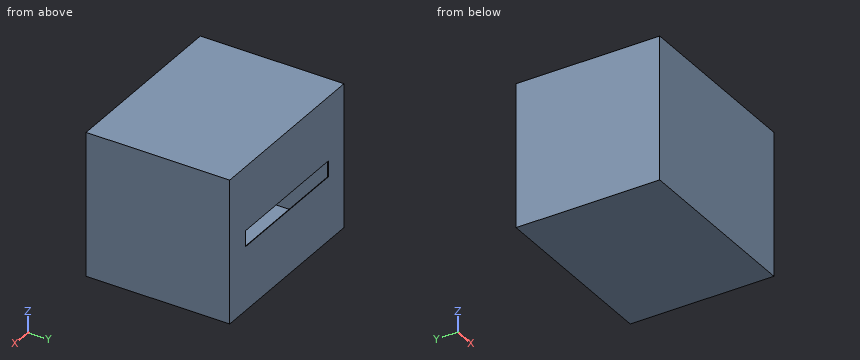
from build123d import *

# Parameters (mm, degrees)
EXTRUDE1_START     = -381
EXTRUDE1_OUTLINE_W = 965.2
EXTRUDE1_OUTLINE_H = 762
EXTRUDE1_DEPTH     = 762
SHELL1_T           = -2.54
SKETCH3_W          = 965.2
SKETCH3_H          = 762
SKETCH3_W_2        = 701.471738738
SKETCH3_H_2        = 84.826616214
EXTRUDE2_DEPTH     = 3.175


# Read off the part's stored shape, not the designer's step: Extrude1
with BuildPart() as part:
    # Extrude1 outline → Extrude1 (new body)
    with BuildSketch(Plane.XY.offset(EXTRUDE1_START)):
        with Locations((482.6, 381)):
            Rectangle(EXTRUDE1_OUTLINE_W, EXTRUDE1_OUTLINE_H)
    extrude(amount=EXTRUDE1_DEPTH)

    # Shell1
    shell1_openings = [part.faces().sort_by_distance(p)[0] for p in [
        (482.6, 762, 0),
    ]]
    offset(amount=SHELL1_T, openings=shell1_openings, kind=Kind.INTERSECTION)

    # Sketch3 → Extrude2 (add)
    with BuildSketch(Plane(origin=(0, 762, 0), x_dir=(-1, 0, 0), z_dir=(0, 1, 0))):
        with Locations((-482.6, 0)):
            Rectangle(SKETCH3_W, SKETCH3_H)
        with Locations((-482.6, 0)):
            Rectangle(SKETCH3_W_2, SKETCH3_H_2, mode=Mode.SUBTRACT)
    extrude(amount=-EXTRUDE2_DEPTH)


solid = part.part
Here's how the part is built. I have some questions about the finished solid (model axes, mm). Round coordinates to 2 decimals unless told otherwise and drop trailing zeros. Order: outer loops, then holes, each group sorted by start corner. A loop starts at its lowest first (then second) coordinate and runs counter-clockwise, first axis right, second up. Notation, with made-up numbers: M 42.25,84 L 75.25,84 A14 cw 75.25,88 Z; hole C 58,76 d2. An arc over 180 degrees is marked long. Return JSON: item names as keys, results as strings. Group by question number.
1. Please list where these lines run through material, in increasing order: probe 1 along Y at (x, z) = (416, -148.5) (3 decimals); probe 2 along Z at (x, y) = (532.5, 206.5); probe 3 along X at (y, z) = (549, 285.5).
2. If we section it at B-B on z = 283.5: List the corners of the cut face in (x, y) for me (3 decimals), then the cut area to 3 significant figures.
3. If we section it at C-C on x = 292: List the corners of the cut face in (y, z) for me (3 decimals).
4. If we section it at A-A on y = 201.5: List the corners of the cut face in (x, z) for me.
Reply:
{
 "1": {"probe 1": "0 to 2.54, 758.825 to 762", "probe 2": "-381 to -378.46, 378.46 to 381", "probe 3": "0 to 2.54, 962.66 to 965.2"},
 "2": {"outline": "M 0,0 L 965.2,0 L 965.2,762 L 0,762 Z; hole M 2.54,2.54 L 962.66,2.54 L 962.66,758.825 L 2.54,758.825 Z", "area": "9,360 mm^2"},
 "3": {"outline": "M 0,-381 L 762,-381 L 762,-42.413 L 758.825,-42.413 L 758.825,-378.46 L 2.54,-378.46 L 2.54,378.46 L 758.825,378.46 L 758.825,42.413 L 762,42.413 L 762,381 L 0,381 Z"},
 "4": {"outline": "M 0,-381 L 965.2,-381 L 965.2,381 L 0,381 Z; hole M 2.54,-378.46 L 962.66,-378.46 L 962.66,378.46 L 2.54,378.46 Z"}
}
